Read the model definition and answer for the solid it produces. Units are mm, in the model's axes. Face numbers are marked on the shaded views. Coordinates: 2 decimals unless noted, no trailing zeros. Write each loop counter-clockwise with the first axis right and the second up, starting at its lowest first coordinate (ties: lowest second). Pieces come first, ordered by that corner, then holes.
from build123d import *

# Parameters (mm, degrees)
F1_DEPTH  = 60
F3_DEPTH  = 3.1
F6_DEPTH  = 3
F8_R      = 1.25
F9_DEPTH  = 100
F10_R     = 1.25
F11_DEPTH = 60


with BuildPart() as f1:
    # F0 (on Right) → F1 (new body)
    with BuildSketch(Plane.YZ):
        Polygon((-4, 0), (0, 0), (10, 0), (10, 4), (10, 82.284271), (-68.284271, 82.284271), (-72.284271, 82.284271), (-72.284271, 72.284271), (-72.284271, 68.284271), (-32.284271, 68.284271), (-7.284271, 68.284271), (-4, 65), (-4, 40), (-4, 8.644639), align=None)
        Polygon((-14, 0), (-4, 0), (-4, 8.644639), (-14, 4), align=None)
    extrude(amount=F1_DEPTH)

    # F2 (on Right) → F3 (join)
    with BuildSketch(Plane.YZ):
        Polygon((-30.521803, 70.845065), (-72.284, 70.845065), (-72.284, 30.845065), (-2.284, 30.845065), (-2.284, 42.845065), (-2.472219, 70.845065), align=None)
    extrude(amount=F3_DEPTH)

    # F5 (on offset) → F6 (join)
    with BuildSketch(Plane.YZ.offset(60)):
        Polygon((-30.521803, 70.845), (-72.284, 70.845), (-72.284, 30.845), (-2.284, 30.845), (-2.284, 42.845), (-2.284, 70.845), align=None)
    extrude(amount=-F6_DEPTH)

    # F8 (on offset) → F9 (cut)
    with BuildSketch(Plane.XZ.offset(25)):
        with Locations((30, 75)):
            Circle(F8_R)
    extrude(amount=F9_DEPTH, mode=Mode.SUBTRACT)

    # F10 (on Top) → F11 (cut)
    with BuildSketch(Plane.XY):
        with Locations((30, 5)):
            Circle(F10_R)
    extrude(amount=F11_DEPTH, mode=Mode.SUBTRACT)


solid = f1.part
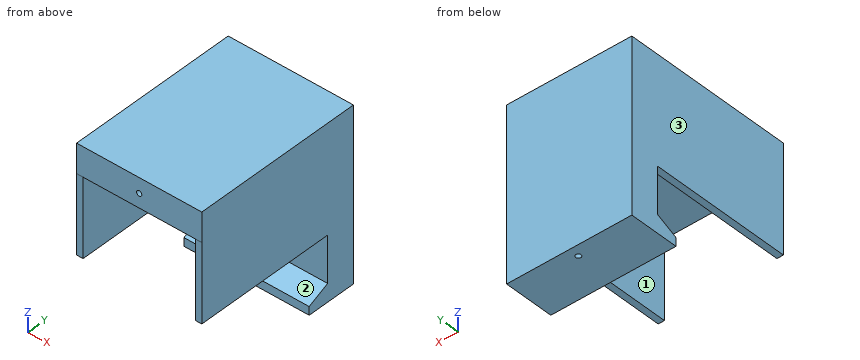
Item 1: Determine the mould class of the marked faces 1, 2 and 3 for opening direction X: +X half, -X half, draft (parallel to the pull), parting line (faces both ways), or undercut.
Item 2: The part is cut by section A-A (z = 41). Give the vertices of the cut face in (x, y), and give its area (3 significant figures).
Item 3: Given pin 1 (17 mm diameter, centred on x = 36, z = 47.5, fed in from -Y); pin 2 (0.9 mm diameter, centred on x = 1, y = -53.5, fed in from -Z); pin 3 (5 mm diameter, centred on x = 40.5, y = -45, fed in from -Z), each flat-ended and moving along its own axis, determine where each tip first touches the part or whether it passes through.
Item 4: The part is cut by section B-B (y = -38). Give the vertices of the cut face in (x, z) (3 decimals), and give its area (3 significant figures).
Item 5: Find the intervals of material crossed by probe 1 along X at (y, z) = (-51, 75); probe 2 along X at (y, z) = (-47.5, 54); probe 3 along Y at (x, z) = (37.5, 60.5), in increasing order.
Item 6: The part is cut by section C-C (y = 5). Give the vertices of the cut face in (x, z).
Item 7: The part is cut by section D-D (x = 30). Give the vertices of the cut face in (y, z).
Answer:
1. face 1: undercut
1. face 2: draft
1. face 3: -X half
2. outline: (0, -72.28) - (3.1, -72.28) - (3.1, -4) - (57, -4) - (57, -72.28) - (60, -72.28) - (60, 10) - (0, 10) - close; hole circle Ø2.5 at (30, 5)
2. area: 1,250 mm2
3. pin 1: stops at y = -4
3. pin 2: stops at z = 30.85
3. pin 3: stops at z = 68.28
4. outline: (0, 30.845) - (3.1, 30.845) - (3.1, 68.284) - (57, 68.284) - (57, 30.845) - (60, 30.845) - (60, 82.284) - (0, 82.284) - close; hole circle Ø2.5 at (30, 75)
4. area: 1,060 mm2
5. probe 1: x = 0 to 28.75, 31.25 to 60
5. probe 2: x = 0 to 3.1, 57 to 60
5. probe 3: y = -4 to 10
6. outline: (0, 0) - (28.75, 0) - (28.75, 60) - (31.25, 60) - (31.25, 0) - (60, 0) - (60, 82.28) - (0, 82.28) - close
7. outline: (-72.28, 68.28) - (-7.28, 68.28) - (-4, 65) - (-4, 8.64) - (-14, 4) - (-14, 0) - (3.75, 0) - (3.75, 60) - (6.25, 60) - (6.25, 0) - (10, 0) - (10, 82.28) - (-72.28, 82.28) - (-72.28, 76.25) - (-25, 76.25) - (-25, 73.75) - (-72.28, 73.75) - close
